CAD build for the part. Positions are in the model's coordinates, mm. Face numbers are marked on the shaded views. A direction names the side the tool comes from. Round coordinates to 2 decimals unless told otherwise and drop trailing zeros. Order: outer loops, then holes, each group sorted by start corner. A loop starts at its lowest first (then second) coordinate and runs counter-clockwise, first axis right, second up. Notation, with made-up numbers: M 81,66.5 L 111,66.5 A30 ccw 111,90.5 Z; hole C 77,51.5 d6. An arc over 180 degrees is marked long. Answer as a JSON object with one key per item and string values.
```python
from build123d import *

# Parameters (mm, degrees)
SKETCH1_W           = 20
SKETCH1_H           = 15
BOSS_EXTRUDE1_DEPTH = 1
SKETCH2_R           = 0.5
CUT_EXTRUDE1_DEPTH  = 1
SKETCH3_R           = 1.5
CUT_EXTRUDE2_DEPTH  = 1
SKETCH4_W           = 5
SKETCH4_H           = 5
BOSS_EXTRUDE2_DEPTH = 1
SKETCH5_W           = 4
SKETCH5_H           = 1
BOSS_EXTRUDE3_DEPTH = 1.5
SKETCH6_W           = 1
SKETCH6_H           = 1.5
BOSS_EXTRUDE4_DEPTH = 1
SKETCH7_W           = 1.379354472
SKETCH7_H           = 1.594878607
SKETCH7_W_2         = 1.853507571
SKETCH7_H_2         = 0.905201372
SKETCH7_W_3         = 1.120725508
SKETCH7_H_3         = 0.646572409
BOSS_EXTRUDE5_DEPTH = 1


with BuildPart() as part:
    # Sketch1 → Boss-Extrude1 (new body)
    with BuildSketch(Plane(origin=(0, 0, 0), x_dir=(1, 0, 0), z_dir=(0, 1, 0))):
        Rectangle(SKETCH1_W, SKETCH1_H)
    extrude(amount=BOSS_EXTRUDE1_DEPTH)

    # Sketch2 → Cut-Extrude1 (cut)
    with BuildSketch(Plane(origin=(0, 1, 0), x_dir=(1, 0, 0), z_dir=(0, 1, 0))):
        with Locations(Location((8.8, 6.5, 0), (0, 0, 270))):
            Circle(SKETCH2_R)
        with Locations(Location((6.3, 6.5, 0), (0, 0, 270))):
            Circle(SKETCH2_R)
        with Locations(Location((3.8, 6.5, 0), (0, 0, 270))):
            Circle(SKETCH2_R)
        with Locations(Location((1.3, 6.5, 0), (0, 0, 270))):
            Circle(SKETCH2_R)
        with Locations(Location((-1.2, 6.5, 0), (0, 0, 270))):
            Circle(SKETCH2_R)
        with Locations(Location((-3.7, 6.5, 0), (0, 0, 270))):
            Circle(SKETCH2_R)
        with Locations(Location((-6.2, 6.5, 0), (0, 0, 270))):
            Circle(SKETCH2_R)
        with Locations(Location((-8.7, 6.5, 0), (0, 0, 270))):
            Circle(SKETCH2_R)
    extrude(amount=-CUT_EXTRUDE1_DEPTH, mode=Mode.SUBTRACT)

    # Sketch3 → Cut-Extrude2 (cut)
    with BuildSketch(Plane(origin=(0, 1, 0), x_dir=(1, 0, 0), z_dir=(0, 1, 0))):
        with Locations(Location((7.909735798, -5.592851334, 0), (0, 0, 270))):
            Circle(SKETCH3_R)
        with Locations(Location((-7.909735798, -5.592851334, 0), (0, 0, 90))):
            Circle(SKETCH3_R)
    extrude(amount=-CUT_EXTRUDE2_DEPTH, mode=Mode.SUBTRACT)

    # Sketch4 → Boss-Extrude2 (add)
    with BuildSketch(Plane(origin=(0, 1, 0), x_dir=(1, 0, 0), z_dir=(0, 1, 0))):
        Rectangle(SKETCH4_W, SKETCH4_H)
    extrude(amount=BOSS_EXTRUDE2_DEPTH)

    # Sketch5 → Boss-Extrude3 (add)
    with BuildSketch(Plane(origin=(0, 1, 0), x_dir=(1, 0, 0), z_dir=(0, 1, 0))):
        with Locations((0, -4.601440307)):
            Rectangle(SKETCH5_W, SKETCH5_H)
    extrude(amount=BOSS_EXTRUDE3_DEPTH)

    # Sketch6 → Boss-Extrude4 (add)
    with BuildSketch(Plane(origin=(0, 1, 0), x_dir=(1, 0, 0), z_dir=(0, 1, 0))):
        with Locations((-6.05193374, 2.062589977)):
            Rectangle(SKETCH6_W, SKETCH6_H)
        with Locations((-4.370845478, 2.062589977)):
            Rectangle(SKETCH6_W, SKETCH6_H)
        with Locations((-6.05193374, -2.062589977)):
            Rectangle(SKETCH6_W, SKETCH6_H)
        with Locations((-4.370845478, -2.062589977)):
            Rectangle(SKETCH6_W, SKETCH6_H)
        with Locations((4.370845478, -2.062589977)):
            Rectangle(SKETCH6_W, SKETCH6_H)
        with Locations((6.05193374, -2.062589977)):
            Rectangle(SKETCH6_W, SKETCH6_H)
        with Locations((4.370845478, 2.062589977)):
            Rectangle(SKETCH6_W, SKETCH6_H)
        with Locations((6.05193374, 2.062589977)):
            Rectangle(SKETCH6_W, SKETCH6_H)
    extrude(amount=BOSS_EXTRUDE4_DEPTH)

    # Sketch7 → Boss-Extrude5 (add)
    with BuildSketch(Plane(origin=(0, 1, 0), x_dir=(1, 0, 0), z_dir=(0, 1, 0))):
        with Locations((-7.888183384, 2.058255501)):
            Rectangle(SKETCH7_W, SKETCH7_H)
        with Locations((7.694211662, 1.260816197)):
            Rectangle(SKETCH7_W_2, SKETCH7_H_2)
        with Locations((8.233022002, 2.381541705)):
            Rectangle(SKETCH7_W_3, SKETCH7_H_3)
        with Locations((8.233022002, 0.140090689)):
            Rectangle(SKETCH7_W_3, SKETCH7_H_3)
    extrude(amount=BOSS_EXTRUDE5_DEPTH)


solid = part.part
```
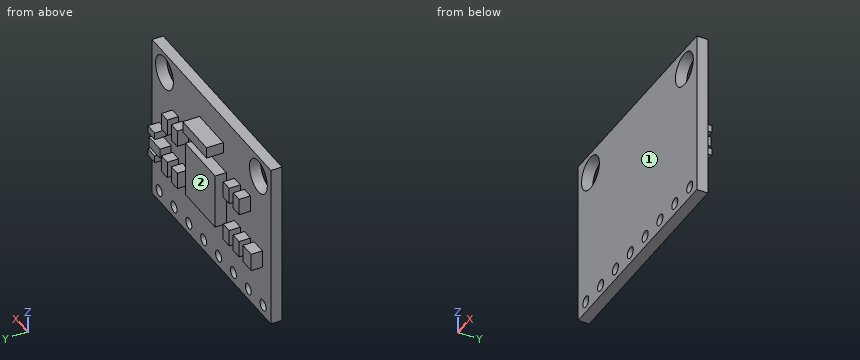
Item 1: Drop flat-ended pins along their axis: pin 1 Ø0.5 at (y, z) = (1.5, -2) entering from +X; pin 2 Ø2.5 at (x, z) = (7.91, 5.59) entering from -Y; pin 3 Ø1.1 at (x, z) = (4.5, 2.5) entering from +Y; pin 4 Ø0.8 at (x, y) = (-4.5, 1.5) entering from -Z. Give the stop position or say it passes through.
Worked answers:
{"pin 1": "stops at x = 8.79", "pin 2": "passes through", "pin 3": "stops at y = 2", "pin 4": "stops at z = -2.81"}
Item 2: Saw through at B-B on y = 0.3. State how many separate pieces and enclosed holes the cut face has, and give its area (3 significant figures).
Worked answers:
{"separate pieces": "1", "enclosed holes": "10", "area": "280 mm2"}
Item 3: 3-axis set-ups, long thin cutter, end or side, ignore diameter. For the marked faces 1 and 2: which of +Z, -Z, +X, -X, +Y, -Y reach the whole face in a straight line?
Worked answers:
{"face 1": "+Z, -Z, +X, -X, -Y", "face 2": "-Z, +X, -X, +Y"}
Item 4: Saw through at A-A on x = -1.2. List the corners of the cut face in (y, z), and give its area (3 significant figures).
Worked answers:
{"outline": "M 0,-7.5 L 1,-7.5 L 1,-7 L 0,-7 Z; M 0,-6 L 1,-6 L 1,-2.5 L 2,-2.5 L 2,2.5 L 1,2.5 L 1,4.1 L 2.5,4.1 L 2.5,5.1 L 1,5.1 L 1,7.5 L 0,7.5 Z", "area": "20.5 mm2"}
Item 5: Wall check: line 1 along X through (y, z) = (0.5, 5.5); line 2 along X through (y, z) = (1.4, -2); line 3 along Z through (x, y) = (1.75, 1.55). Give the ranges that are in metal, low to high. Write a range as [from, to].
Worked answers:
{"line 1": "x = [-10, -9.41], [-6.41, 6.41], [9.41, 10]", "line 2": "x = [-8.58, -7.2], [-6.55, -5.55], [-4.87, -3.87], [-2.5, 2.5], [3.87, 4.87], [5.55, 6.55]", "line 3": "z = [-2.5, 2.5], [4.1, 5.1]"}
